```python
from build123d import *

# Parameters (mm, degrees)
F0_W     = 50.7999993861
F0_H     = 50.8000031114
F1_DEPTH = 50.8
F2_SIZE  = 5.08


with BuildPart() as f1:
    # F0 (on Front) → F1 (new body)
    with BuildSketch(Plane.XZ):
        with Locations((25.399999693, 25.4000015557)):
            Rectangle(F0_W, F0_H)
    extrude(amount=F1_DEPTH)

    # F2
    f2_edges = [f1.edges().sort_by_distance(p)[0] for p in [
        (25.4, -50.8, 50.800003),
        (0, -50.8, 25.400002),
        (25.4, -50.8, 0),
        (50.799999, -50.8, 25.400002),
        (50.799999, -25.4, 50.800003),
        (25.4, 0, 50.800003),
        (0, -25.4, 50.800003),
        (0, 0, 25.400002),
        (25.4, 0, 0),
        (50.799999, 0, 25.400002),
        (0, -25.4, 0),
        (50.799999, -25.4, 0),
    ]]
    chamfer(f2_edges, length=F2_SIZE)

    # F3 (on face) → F4 (revolve, cut)
    with BuildSketch(Plane(origin=(0, 0, 0), x_dir=(-1, 0, 0), z_dir=(0, 1, 0))):
        with BuildLine():
            Line((-25.399999693, 28.2762738749), (-25.399999693, 22.5237292365))
            ThreePointArc((-25.399999693, 22.5237292365), (-23.3661680316, 23.3661698942), (-22.5237273738, 25.4000015557))
            ThreePointArc((-22.5237273738, 25.4000015557), (-23.3661680316, 27.4338332171), (-25.399999693, 28.2762738749))
        make_face()
    revolve(axis=Axis((25.399999693, 0, 25.4000015557), (0, 0, 1)), mode=Mode.SUBTRACT)

    # F5 (on face) → F6 (revolve, cut)
    with BuildSketch(Plane.XY.offset(50.8000031114)):
        with BuildLine():
            Line((33.7353862623, -33.6240240537), (37.8023569838, -37.6751894799))
            ThreePointArc((37.8023569838, -37.6751894799), (38.4216586219, -36.745402906), (38.639071623, -35.6496067668))
            ThreePointArc((38.639071623, -35.6496067668), (36.8646677623, -32.9968197679), (33.7353862623, -33.6240240537))
        make_face()
        with BuildLine():
            ThreePointArc((18.8353189816, -15.9228166067), (17.0609151208, -13.2700296079), (13.9316336208, -13.8972338936))
            Line((13.9316336208, -13.8972338936), (17.9986043423, -17.9483993198))
            ThreePointArc((17.9986043423, -17.9483993198), (18.6179059804, -17.018612746), (18.8353189816, -15.9228166067))
        make_face()
    revolve(axis=Axis((25.2446672624, -25.1663021739, 50.8000031114), (-0.708482113, 0.7057287691, 0)), mode=Mode.SUBTRACT)

    # F7 (on face) → F8 (revolve, cut)
    with BuildSketch(Plane.YZ.offset(50.7999993861)):
        with BuildLine():
            ThreePointArc((-32.9918336927, 35.8620360494), (-34.7636556544, 38.5137550626), (-37.8915714984, 37.8915740104))
            Line((-37.8915714984, 37.8915740104), (-33.832495887, 33.8324980883))
            ThreePointArc((-33.832495887, 33.8324980883), (-33.2103146795, 34.763658011), (-32.9918336927, 35.8620360494))
        make_face()
        with BuildLine():
            ThreePointArc((-22.5298, 25.4000015557), (-24.3016219617, 28.0517205689), (-27.4295378057, 27.4295395167))
            Line((-27.4295378057, 27.4295395167), (-23.3704621943, 23.3704635946))
            ThreePointArc((-23.3704621943, 23.3704635946), (-22.7482809868, 24.3016235174), (-22.5298, 25.4000015557))
        make_face()
        with BuildLine():
            Line((-15.8805371302, 15.8805379571), (-11.8214615189, 11.821462035))
            ThreePointArc((-11.8214615189, 11.821462035), (-11.1992803114, 12.7526219577), (-10.9807993246, 13.8509999961))
            ThreePointArc((-10.9807993246, 13.8509999961), (-12.7526212862, 16.5027190093), (-15.8805371302, 15.8805379571))
        make_face()
    revolve(axis=Axis((50.7999993861, -25.4, 25.4000015557), (0, 0.7071067541, -0.7071068083)), mode=Mode.SUBTRACT)


solid = f1.part
```
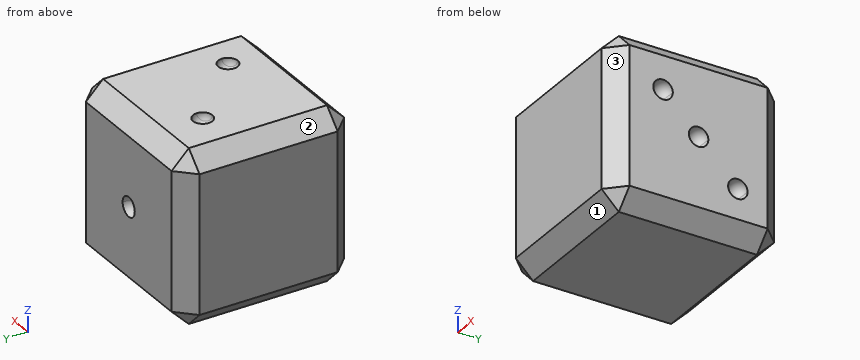
Design review of the part built by this model. Coordinates are the model's own, in mm. Face numbers are marked on the shaded views. Give positions to 0.01 mm unless a question says otherwise; leave off trailing zeros. Write each loop counter-clockwise with the first axis right and the second up, starting at its lowest first coordinate (ties: lowest second). Pieces come first, ordered by that corner, then holes.
(1) Clearance check with a flat-ended pin moving along its axis: pin 1 Ø5 at (x, y) = (17, -14) entering from +Z. State where the tip first meets the part, or that it passes through.
Checked values:
pin 1: stops at z = 50.8
(2) Wall thickness on line 1 along Y through (x, z) = (16.5, 48.5); line 2 along Y through (x, z) = (47.5, 44.5); line 3 along X through (y, z) = (-4, 45.5): over which ranges is each line inside the solid? List them lowest first.
Checked values:
line 1: y = -48.02 to -17.55, -14.29 to -2.78
line 2: y = -49.02 to -1.78
line 3: x = 1.08 to 49.72
(3) Add section A-A (z = 46.5). Give the boundary of the cut face in (x, y), and give its area (3 significant figures).
Checked values:
outline: (0.78, -45.72) - (5.08, -50.02) - (45.72, -50.02) - (50.02, -45.72) - (50.02, -5.08) - (45.72, -0.78) - (5.08, -0.78) - (0.78, -5.08) - close
area: 2,390 mm2
(4) Mouldability with a two-part tool opening along Z and no side actions: class the marked faces 1, 2 and 3 as +Z half, -Z half, draft (parallel to the pull), parting line (faces both ways), or undercut.
Checked values:
face 1: -Z half
face 2: +Z half
face 3: draft
(5) Add section B-B (y = -29.5). Give the boundary of the cut face in (x, z).
Checked values:
outline: (0, 5.08) - (5.08, 0) - (45.72, 0) - (50.8, 5.08) - (50.8, 45.72) - (45.72, 50.8) - (5.08, 50.8) - (0, 45.72) - close
(6) Add section C-C (x = 27). Give the boundary of the cut face in (y, z), and give its area (3 significant figures).
Checked values:
outline: (-50.8, 5.08) - (-45.72, 0) - (-5.08, 0) - (0, 5.08) - (0, 23.01) arc R2.39 cw to (0, 27.79) - (0, 45.72) - (-5.08, 50.8) - (-45.72, 50.8) - (-50.8, 45.72) - close
area: 2,520 mm2
(7) Add section D-D (z = 37). Give the boundary of the cut face in (x, y), and give its area (3 significant figures).
Checked values:
outline: (0, -45.72) - (5.08, -50.8) - (45.72, -50.8) - (50.8, -45.72) - (50.8, -38.5) arc R2.63 cw to (50.8, -33.23) - (50.8, -5.08) - (45.72, 0) - (5.08, 0) - (0, -5.08) - close
area: 2,520 mm2
